Verification items for the finished model (mm, model axes). Give positions to 0.01 mm unless a question says otherwise; leave off trailing zeros. Loops run counter-clockwise (first coordinate to the right, second up) from the corner with the lowest first, then second, coordinate; pieces in that order, holes last. Notation, with made-up numbers: (6, 19) - (41, 19) arc R34 cw to (41, 53) - close; hole circle Ø11 at (-19.5, 89.5). An arc over 180 degrees is marked (long way). One line per item, written item: value. Start each with the question number.
1. Sectioned sample at A-A (y = 5). Record the cut outline in (x, z), plus the area to 3 significant figures.
2. Scan lines: L1, parallel to Y at x = 15, z = 0.4; L2, parallel to Y at x = 12.75, z = 0.8; L3, parallel to Y at x = 13.8, z = 1.15. Record each from-to range of solid material in increasing order. Write a range as [from, to].
3. Sectioned sample at D-D (x = 13.8). Record the cut outline in (y, z).
4. Sectioned sample at B-B (y = 24.1). Record the cut outline in (x, z).
5. Sectioned sample at C-C (x = 7). Record the cut outline in (y, z).
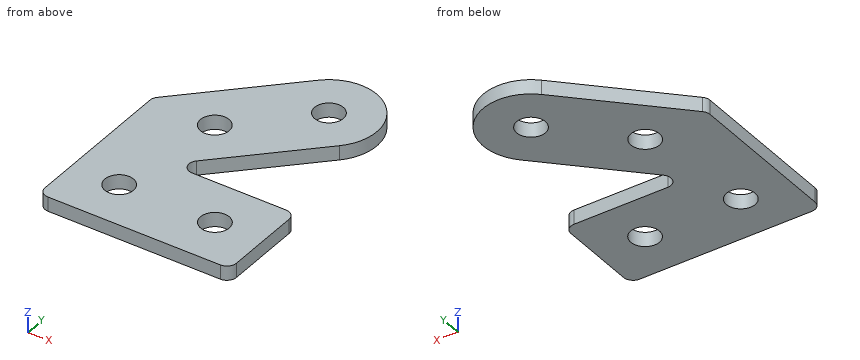
from build123d import *

# Parameters (mm, degrees)
SCHIZZO1_W                   = 20
SCHIZZO1_H                   = 10
ESTRUSIONE_ESTRUSIONE1_DEPTH = 1.5
FORO_3_0_3_1_D               = 3
ESTRUSIONE_ESTRUSIONE3_DEPTH = 1.5
FORO_3_0_3_4_D               = 3
RACCORDO2_R                  = 1


with BuildPart() as part:
    # Schizzo1 → Estrusione-Estrusione1 (new body)
    with BuildSketch(Plane.XY):
        with Locations((10, 5)):
            Rectangle(SCHIZZO1_W, SCHIZZO1_H)
    extrude(amount=ESTRUSIONE_ESTRUSIONE1_DEPTH)

    # Foro Ø3.0 (3)-1 (through all)
    with Locations(Plane.XY.offset(1.5)):
        with Locations((5, 5), (15, 5)):
            Hole(FORO_3_0_3_1_D / 2)

    # Schizzo9 → Estrusione-Estrusione3 (add)
    with BuildSketch(Plane.XY):
        with BuildLine():
            Line((0, 17.371067812), (0, 10))
            Line((0, 10), (6.771067812, 10))
            Line((6.771067812, 10), (17.335533906, 20.564466094))
            ThreePointArc((17.335533906, 20.564466094), (17.335533906, 27.635533906), (10.264466094, 27.635533906))
            Line((10.264466094, 27.635533906), (0, 17.371067812))
        make_face()
    extrude(amount=ESTRUSIONE_ESTRUSIONE3_DEPTH)

    # Foro Ø3.0 (3)-4 (through all)
    with Locations(Plane.XY.offset(1.5)):
        with Locations((13.8, 24.1), (6.728932188, 17.028932188)):
            Hole(FORO_3_0_3_4_D / 2)

    # Raccordo2
    raccordo2_edges = [part.edges().sort_by_distance(p)[0] for p in [
        (0, 0, 0.75),
        (20, 0, 0.75),
        (20, 10, 0.75),
        (6.771067812, 10, 0.75),
        (0, 17.371067812, 0.75),
    ]]
    fillet(raccordo2_edges, radius=RACCORDO2_R)


solid = part.part
Results are:
1. outline: (0, 0) - (3.5, 0) - (3.5, 1.5) - (0, 1.5) - close; (6.5, 0) - (13.5, 0) - (13.5, 1.5) - (6.5, 1.5) - close; (16.5, 0) - (20, 0) - (20, 1.5) - (16.5, 1.5) - close
1. area: 21.0 mm^2
2. L1: y = [0, 3.5], [6.5, 10], [18.23, 23.2], [25, 28.95]
2. L2: y = [0, 10], [15.98, 23.03], [25.17, 28.99]
2. L3: y = [0, 4.1], [5.9, 10], [17.03, 22.6], [25.6, 29.1]
3. outline: (0, 0) - (4.1, 0) - (4.1, 1.5) - (0, 1.5) - close; (5.9, 0) - (10, 0) - (10, 1.5) - (5.9, 1.5) - close; (17.03, 0) - (22.6, 0) - (22.6, 1.5) - (17.03, 1.5) - close; (25.6, 0) - (29.1, 0) - (29.1, 1.5) - (25.6, 1.5) - close
4. outline: (6.73, 0) - (12.3, 0) - (12.3, 1.5) - (6.73, 1.5) - close; (15.3, 0) - (18.8, 0) - (18.8, 1.5) - (15.3, 1.5) - close
5. outline: (0, 0) - (15.55, 0) - (15.55, 1.5) - (0, 1.5) - close; (18.5, 0) - (24.37, 0) - (24.37, 1.5) - (18.5, 1.5) - close
